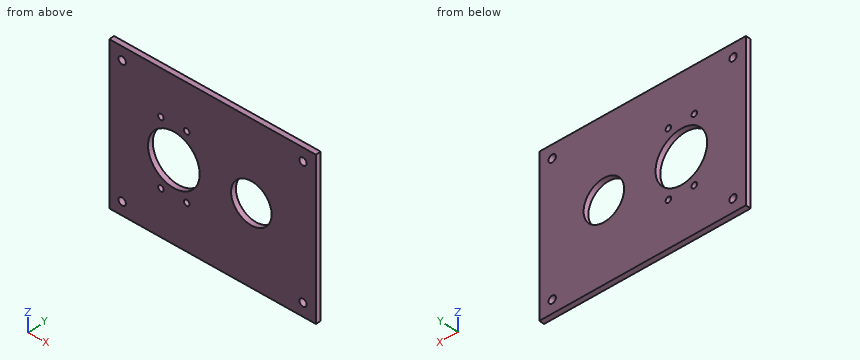
from build123d import *

# Parameters (mm, degrees)
SKETCH1_W           = 240
SKETCH1_H           = 180
SKETCH1_R           = 23.55
SKETCH1_R_2         = 30
SKETCH1_R_3         = 4.25
SKETCH1_R_4         = 3.25
PLATE_EXTRUDE_DEPTH = 6


with BuildPart() as part:
    # Sketch1 → Plate_Extrude (new body)
    with BuildSketch(Plane(origin=(0, 0, 0), x_dir=(1, 0, 0), z_dir=(0, 1, 0))):
        Rectangle(SKETCH1_W, SKETCH1_H)
        with Locations(Location((45, 0, 0), (0, 0, 270))):
            Circle(SKETCH1_R, mode=Mode.SUBTRACT)
        with Locations(Location((-45, 0, 0), (0, 0, 270))):
            Circle(SKETCH1_R_2, mode=Mode.SUBTRACT)
        with Locations(Location((-105, -75, 0), (0, 0, 270))):
            Circle(SKETCH1_R_3, mode=Mode.SUBTRACT)
        with Locations(Location((105, -75, 0), (0, 0, 270))):
            Circle(SKETCH1_R_3, mode=Mode.SUBTRACT)
        with Locations(Location((-105, 75, 0), (0, 0, 270))):
            Circle(SKETCH1_R_3, mode=Mode.SUBTRACT)
        with Locations(Location((105, 75, 0), (0, 0, 270))):
            Circle(SKETCH1_R_3, mode=Mode.SUBTRACT)
        with Locations(Location((-60, -38, 0), (0, 0, 270))):
            Circle(SKETCH1_R_4, mode=Mode.SUBTRACT)
        with Locations(Location((-60, 38, 0), (0, 0, 270))):
            Circle(SKETCH1_R_4, mode=Mode.SUBTRACT)
        with Locations(Location((-30, -38, 0), (0, 0, 270))):
            Circle(SKETCH1_R_4, mode=Mode.SUBTRACT)
        with Locations(Location((-30, 38, 0), (0, 0, 270))):
            Circle(SKETCH1_R_4, mode=Mode.SUBTRACT)
    extrude(amount=PLATE_EXTRUDE_DEPTH)


solid = part.part
Check sheet for the modelled part. Datum: model origin and axes. Units: mm. Round coordinates to 2 decimals unless told otherwise and drop trailing zeros. Order: outer loops, then holes, each group sorted by start corner. A loop starts at its lowest first (then second) coordinate and runs counter-clockwise, first axis right, second up. Notation, with made-up numbers: M 37,59.25 L 55,59.25 A32 cw 55,88.25 Z; hole C -5,74 d10. An arc over 180 degrees is marked long. One line per item, written item: value. Start each with the question number.
1. Gauge pin test, flat end, axial feed: P1, Ø10.5, axis at x = -60, z = -38, coming from the -Y side. Record the tip position at first contact, or that the pin passes through.
2. Section check D-D on x = -60. Enter the section's corners in (y, z), and give its area (3 significant figures).
3. Section check B-B on z = 0. Enter the section's corners in (x, y), and give its area (3 significant figures).
4. Section check A-A on x = 105. Enter the section's corners in (y, z).
5. Section check C-C on y = 4.1. Give the number of separate pieces and of enclosed holes in the cut face, and give its area (3 significant figures).
6. Scan lines: line 1 along X through (y, z) = (4.75, -38); line 2 along X through (y, z) = (4.5, 0); line 3 along Z through (x, y) = (43.5, 1.4). Record each from-to range of solid material in increasing order.
Results found:
1. P1: y = 0
2. outline: M 0,-90 L 6,-90 L 6,-41.25 L 0,-41.25 Z; M 0,-34.75 L 6,-34.75 L 6,-25.98 L 0,-25.98 Z; M 0,25.98 L 6,25.98 L 6,34.75 L 0,34.75 Z; M 0,41.25 L 6,41.25 L 6,90 L 0,90 Z
2. area: 690 mm^2
3. outline: M -120,0 L -75,0 L -75,6 L -120,6 Z; M -15,0 L 21.45,0 L 21.45,6 L -15,6 Z; M 68.55,0 L 120,0 L 120,6 L 68.55,6 Z
3. area: 797 mm^2
4. outline: M 0,-90 L 6,-90 L 6,-79.25 L 0,-79.25 Z; M 0,-70.75 L 6,-70.75 L 6,70.75 L 0,70.75 Z; M 0,79.25 L 6,79.25 L 6,90 L 0,90 Z
5. separate pieces: 1
5. enclosed holes: 10
5. area: 38,300 mm^2
6. line 1: -120 to -63.25, -56.75 to -33.25, -26.75 to 120
6. line 2: -120 to -75, -15 to 21.45, 68.55 to 120
6. line 3: -90 to -23.5, 23.5 to 90
